Geometry: see drawing. Coordinates: mm, zero at the bounding-box minimum. A direction names the side the tool comes from. Coordinates: 2 decimals unless noted, no trailing zeros. Loops run counter-clockwise (first coordinate to the right, second up) from the corner with the lowest first, then second, coordinate; pieces in that order, holes last. Notation, with made-up numbers: (12.25, -25.5) -> (60.25, -25.5) arc R10 cw to (60.25, -19.5) -> close; hole circle Ø10 at (21, 42.5). An arc over 180 degrees is marked (long way). Put each result on its own line as item: value. Start each with the question number.
1) Cut plane C-C (z = 0.75). Return the cut outline in (x, y).
2) Contact query for flat-ended pins moving along their axis: P1, Ø0.9, axis at x = 15.5, z = 1.5, coming from the -Y side; P2, Ø2, axis at x = 5.5, y = 16.5, coming from the -Z side; P3, Ø1.5, axis at x = 15.5, z = 2, coming from the +Y side. Output: stop coordinate, or through.
3) Set-up query: the marked faces 1 and 2. Return all of +Z, -Z, +X, -X, +Y, -Y with unobstructed straight access to the full face (end or side cutting, diameter ignored); none if empty.
4) Material intervals for L1, parallel to Z at x = 11, y = 13.5 (1 decimal); L2, parallel to Z at x = 16.5, y = 34; L3, parallel to Y at x = 12.5, z = 2.3, sorted ascending.
5) Cut plane B-B (x = 31). Return the cut outline in (y, z).
6) Cut plane A-A (y = 22). Return the cut outline in (x, z).
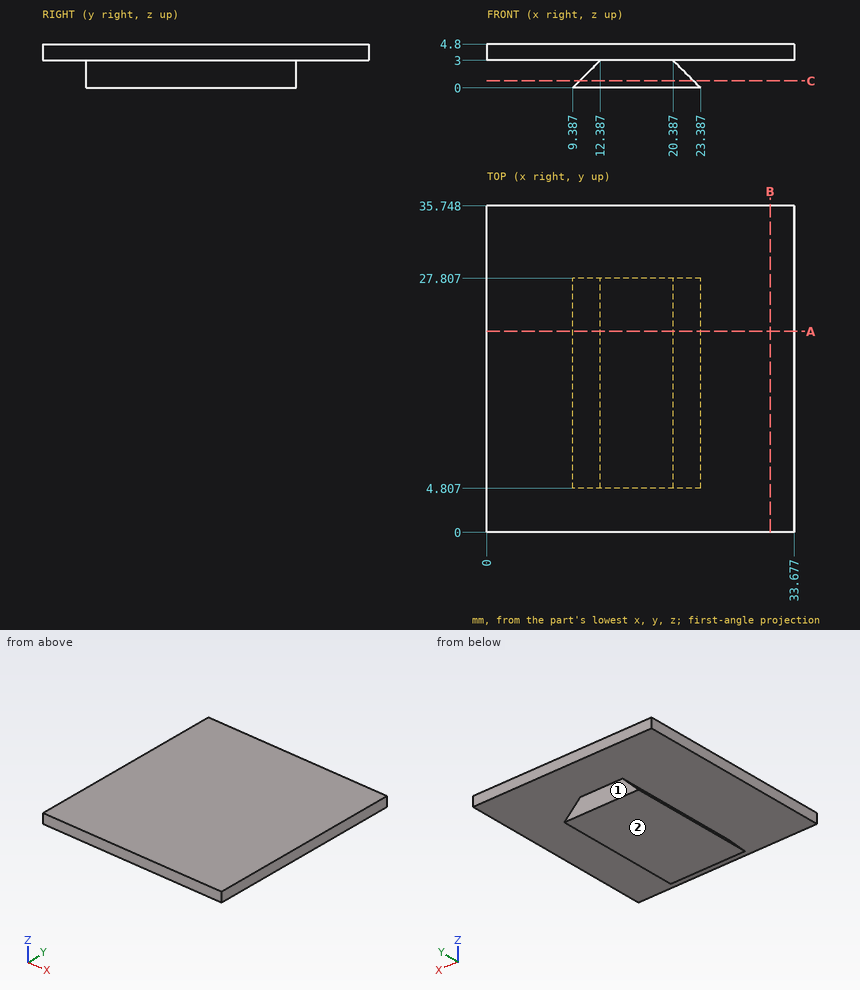
Results found:
1. outline: (10.14, 4.81) -> (22.64, 4.81) -> (22.64, 27.81) -> (10.14, 27.81) -> close
2. P1: stops at y = 4.81
2. P2: stops at z = 3
2. P3: stops at y = 27.81
3. face 1: -Z, +X, -X, +Y
3. face 2: -Z, +X, -X, +Y, -Y
4. L1: z = 0 to 1.6, 3 to 4.8
4. L2: z = 3 to 4.8
4. L3: y = 4.81 to 27.81
5. outline: (0, 3) -> (35.75, 3) -> (35.75, 4.8) -> (0, 4.8) -> close
6. outline: (0, 3) -> (12.39, 3) -> (9.39, 0) -> (23.39, 0) -> (20.39, 3) -> (33.68, 3) -> (33.68, 4.8) -> (0, 4.8) -> close
